```python
from build123d import *

# Parameters (mm, degrees)
SKETCH_1_R          = 5
SKETCH_1_R_2        = 4
EXTRUDE_1_DEPTH     = 220
SKETCH_2_R          = 1.7
CUT_EXTRUDE_1_DEPTH = 10
CUT_EXTRUDE_START   = 16
SKETCH_3_R          = 1.7
CUT_EXTRUDE_3_DEPTH = 16


with BuildPart() as part:
    # 草图1 → 拉伸1 (new body)
    with BuildSketch(Plane.XY):
        Circle(SKETCH_1_R)
        Circle(SKETCH_1_R_2, mode=Mode.SUBTRACT)
    extrude(amount=EXTRUDE_1_DEPTH)

    # 草图2 → 切除-拉伸1 (cut)
    with BuildSketch(Plane(origin=(0, 0, 0), x_dir=(1, 0, 0), z_dir=(0, 1, 0))):
        with Locations(Location((0, -5, 0), (0, 0, 270))):
            Circle(SKETCH_2_R)
        with BuildLine():
            Line((-2, -210), (-2, -20))
            ThreePointArc((-2, -20), (0, -18), (2, -20))
            Line((2, -20), (2, -210))
            ThreePointArc((2, -210), (0, -212), (-2, -210))
        make_face()
    extrude(amount=-CUT_EXTRUDE_1_DEPTH, mode=Mode.SUBTRACT)

    # 草图3 → 切除-拉伸3 (cut)
    with BuildSketch(Plane(origin=(0, 0, 0), x_dir=(1, 0, 0), z_dir=(0, 1, 0)).offset(CUT_EXTRUDE_START)):
        with Locations(Location((0, -5, 0), (0, 0, 270))):
            Circle(SKETCH_3_R)
    extrude(amount=-CUT_EXTRUDE_3_DEPTH, mode=Mode.SUBTRACT)


solid = part.part
```
Model file for the job. Use its own axes, mm. Give positions to 0.01 mm unless a question says otherwise; leave off trailing zeros. Order: outer loops, then holes, each group sorted by start corner. A loop starts at its lowest first (then second) coordinate and runs counter-clockwise, first axis right, second up.
1) Saw through at C-C, the plane z = 16. Write the cut outline in (x, y), then the cut area to 3 significant figures.
2) Pin check, flat tips, straight feed: pin 1 (1.5 mm diameter, centred on x = -0.5, z = 194.5, fed in from -Y); pin 2 (1 mm diameter, centred on x = -2.5, z = 160.5, fed in from +Y); pin 3 (0.6 mm diameter, centred on y = -4, z = 79, fed in from -X). Stop position of each tip, or through.
3) Saw through at B-B, the plane y = 0. Write the cut outline in (x, z).
4) Wall check: probe 1 along Z at (x, y) = (0, -4.45); probe 2 along Z at (x, y) = (0, 4.7); probe 3 along X at (y, z) = (-2.25, 11.5). Give the ranges that are in metal, low to high.
5) Saw through at D-D, the plane z = 179. Write the cut outline in (x, y).
6) Mould opens along X. For faces 1 (the cylindrical face through (3, 4, 108)), 2 (the cylindrical face through (-0.521, 3.966, 108.46)), 3 (the cylindrical face through (0.51, -4.3, 6.62)) say: +X half, -X half, draft (parallel to the pull), parting line (faces both ways), or undercut.
7) Saw through at A-A, the plane x = 0. Write the cut outline in (y, z).
Computed:
1. outline: circle Ø10 at (0, 0); hole circle Ø8 at (0, 0)
1. area: 28.3 mm2
2. pin 1: stops at y = 3.8
2. pin 2: stops at y = 4.58
2. pin 3: stops at x = -3.36
3. outline: (-5, 0) - (-4, 0) - (-4, 220) - (-5, 220) - close; (4, 0) - (5, 0) - (5, 220) - (4, 220) - close
4. probe 1: z = 0 to 3.3, 6.7 to 18, 212 to 220
4. probe 2: z = 0 to 3.3, 6.7 to 220
4. probe 3: x = -4.47 to -3.31, 3.31 to 4.47
5. outline: (-2, -4.58) - (-2, -3.46) arc R4 cw (long way) to (2, -3.46) - (2, -4.58) arc R5 ccw (long way) to start
6. face 1: parting line
6. face 2: undercut
6. face 3: undercut
7. outline: (-5, 0) - (-4, 0) - (-4, 3.3) - (-5, 3.3) - close; (-5, 6.7) - (-4, 6.7) - (-4, 18) - (-5, 18) - close; (-5, 212) - (-4, 212) - (-4, 220) - (-5, 220) - close; (4, 0) - (5, 0) - (5, 3.3) - (4, 3.3) - close; (4, 6.7) - (5, 6.7) - (5, 220) - (4, 220) - close
